Can you work these out from the drawing? Everything is in mm from the part's minimum corner. A direction names the side the tool comes from. Coordinates: 2 decimals unless noted, no trailing zeros. Order: outer loops, then holes, each group sorted by start corner. A loop starts at its lowest first (then second) coordinate and runs counter-clockwise, first axis right, second up. Notation, with made-up numbers: (-33, 87) -> (11, 87) arc R30 cw to (11, 125) -> close; hole circle Ø5 at (-36.75, 20.5). An arc over 180 degrees is marked (long way). Put each result on its own line as item: value. Start each with the question number.
Q1. If we section it at B-B (y = 4): Please give me the cut outline in (x, z), and give its area (3 significant figures).
Q2. If we section it at C-C (z = 10.75): Please give me the cut outline in (x, y).
Q3. For the marked faces 1, 2, 3, 4 and 5, which set-ups out of +Z, -Z, +X, -X, +Y, -Y let a thin tool reach every point of the face, with its end or its side?
Q4. We'd pull the mould along X, two halves only. Please class the marked faces 6, 7 and 8: +X half, -X half, draft (parallel to the pull), parting line (faces both ways), or undercut.
Q5. Please list where these lines run through material, in increasing order: line 1 along Z through (x, y) = (4, 3.5); line 2 along Y through (x, z) = (25, 5.5); line 3 along X through (y, z) = (27, 4).
Q6. If we section it at A-A (x = 4): Please give me the cut outline in (y, z).
Q7. If we section it at D-D (y = 24.5): Please give me the cut outline in (x, z).
Q8. Will these pins go through, and if not, where does the flat tip stop? pin 1 (1.5 mm diameter, centred on y = 20, z = 3, fed in from +X); pin 2 (2.5 mm diameter, centred on x = 46.5, z = 6.5, fed in from +Y); pin 3 (4.5 mm diameter, centred on y = 24.5, z = 7.5, fed in from -X).
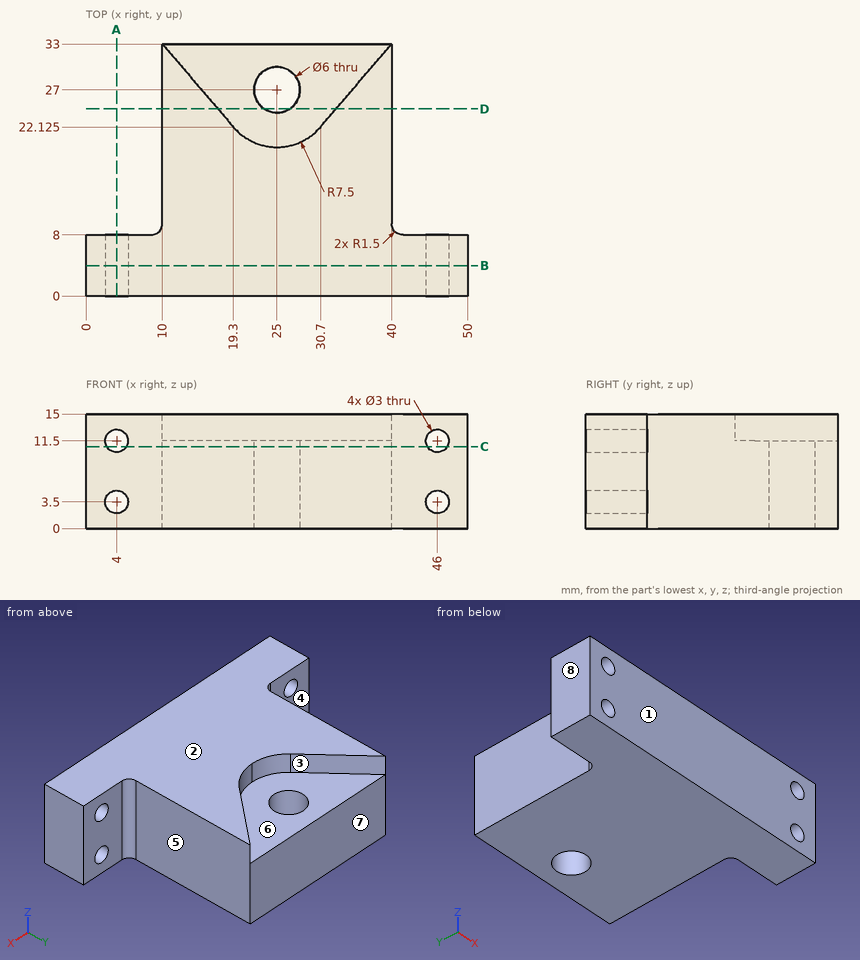
The answers:
1. outline: (0, 0) -> (50, 0) -> (50, 15) -> (0, 15) -> close; hole circle Ø3 at (4, 3.5); hole circle Ø3 at (4, 11.5); hole circle Ø3 at (46, 3.5); hole circle Ø3 at (46, 11.5)
1. area: 722 mm^2
2. outline: (0, 0) -> (2.7, 0) -> (2.7, 8) -> (0, 8) -> close; (5.3, 0) -> (44.7, 0) -> (44.7, 8) -> (41.5, 8) arc R1.5 cw to (40, 9.5) -> (40, 33) -> (10, 33) -> (10, 9.5) arc R1.5 cw to (8.5, 8) -> (5.3, 8) -> close; (47.3, 0) -> (50, 0) -> (50, 8) -> (47.3, 8) -> close; hole circle Ø6 at (25, 27)
3. face 1: +Z, -Z, +X, -X, -Y
3. face 2: +Z, +X, -X, +Y, -Y
3. face 3: +Z, +Y
3. face 4: +Z, -Z, -X, +Y
3. face 5: +Z, -Z, +X, +Y
4. face 6: undercut
4. face 7: draft
4. face 8: -X half
5. line 1: 0 to 2, 5 to 10, 13 to 15
5. line 2: 0 to 24, 30 to 33
5. line 3: 10 to 22, 28 to 40
6. outline: (0, 0) -> (8, 0) -> (8, 2) -> (0, 2) -> close; (0, 5) -> (8, 5) -> (8, 10) -> (0, 10) -> close; (0, 13) -> (8, 13) -> (8, 15) -> (0, 15) -> close
7. outline: (10, 0) -> (23.34, 0) -> (23.34, 11.5) -> (17.27, 11.5) -> (17.27, 15) -> (10, 15) -> close; (26.66, 0) -> (40, 0) -> (40, 15) -> (32.73, 15) -> (32.73, 11.5) -> (26.66, 11.5) -> close
8. pin 1: x = 40
8. pin 2: y = 8
8. pin 3: x = 10
